Read the model definition and answer for the solid it produces. Units are mm, in the model's axes. A direction names the side the tool comes from. Give positions to 0.01 mm unless a question says otherwise; leave off trailing zeros. Order: outer loops, then holes, each group sorted by start corner. A loop starts at its lowest first (then second) coordinate and runs counter-clockwise, first axis right, second up. Notation, with made-up numbers: (38, 15.5) -> (88, 15.5) arc R23 cw to (88, 52.5) -> close; hole circle Ø5 at (60.25, 12.25). An arc over 180 degrees is marked (long way). Answer as CSV lines item,"result". Start each with the question number.
1) Straight lines are drawn through the part: L1, parallel to X at y = 7, z = -40; L2, parallel to X at y = 10, z = 10.25; L3, parallel to X at y = 1, z = -5. For each, find the intervals that lie inside material, in ascending order. Write a range as from..to.
2) Find section D-D (z = 7). Determine the outline of the cut face in (x, y), and give its area (3 significant figures).
3) The mould has two halves that part along Z. Classify faces 4 (the face through (82.4, 10.1, 8.2)), 5 (the face through (10, 70, 11.46)), 6 (the face through (62, 28, 5)), 7 (the face through (97, 5, -4)): +Z half, -Z half, draft (parallel to the pull), parting line (faces both ways), or undercut.
4) Find section A-A (z = -5). Determine the outline of the cut face in (x, y).
5) For faces 1 (the face through (3.659, 19.344, -1.767)), 2 (the face through (97, 2, -25)), 3 (the face through (87, 28, 5)), determine the directions among +Z, -Z, +X, -X, +Y, -Y from which every point of the face is accessible in a straight line to the end or side of a thin tool.
6) Find section B-B (x = 85). State how many separate pieces and enclosed holes the cut face has, and give its area (3 significant figures).
7) Flat-ended cylindrical pins translate along their axes: pin 1 Ø10 at (x, z) = (53, -17.5) entering from +Y; pin 2 Ø4 at (x, y) = (98, 3) entering from -Z; pin 3 Ø10 at (x, y) = (59.5, 28) entering from -Z. Find the tip coordinate at first contact, or state that the pin passes through.
```python
from build123d import *

# Parameters (mm, degrees)
BOSS_EXTRUDE1_DEPTH     = 10
SKETCH2_R               = 2.6
CUT_EXTRUDE1_DEPTH      = 142.774468788
BOSS_EXTRUDE3_START     = 10
SKETCH3_W               = 60
SKETCH3_H               = 9
SKETCH3_W_2             = 9
SKETCH3_H_2             = 60
BOSS_EXTRUDE3_DEPTH     = 1.46
CUT_EXTRUDE2_DEPTH      = 142.884923794
CUT_EXTRUDE2_DEPTH_BACK = 142.884923794
SKETCH2_2_R             = 2.6
CHAMFER1_SIZE           = 1.46
SKETCH4_R               = 4.5
CUT_EXTRUDE3_DEPTH      = 5
SKETCH5_W               = 100
SKETCH5_H               = 50
BOSS_EXTRUDE4_DEPTH     = 5
BOSS_EXTRUDE5_DEPTH     = 10
BOSS_EXTRUDE6_START     = 100
BOSS_EXTRUDE6_DEPTH     = 10
CUT_EXTRUDE4_DEPTH      = 151
CUT_EXTRUDE4_DEPTH_BACK = 151
SKETCH10_R              = 1.75
CUT_EXTRUDE5_START      = 100
SKETCH11_R              = 3.5
CUT_EXTRUDE5_DEPTH      = 95
SKETCH12_W              = 5
SKETCH12_H              = 10
SKETCH12_W_2            = 10
SKETCH12_H_2            = 5
CUT_EXTRUDE6_DEPTH      = 5
CHAMFER2_SIZE           = 5


# Some blends are built 0.0001 mm under size
with BuildPart() as part:
    # Sketch1 → Boss-Extrude1 (new body)
    with BuildSketch(Plane.XY):
        Polygon((0, 0), (100, 0), (100, 40), (20, 100), (0, 100), align=None)
    extrude(amount=BOSS_EXTRUDE1_DEPTH)

    # Sketch2 → Cut-Extrude1 (cut, through all)
    with BuildSketch(Plane.XY):
        with Locations((10, 85)):
            Circle(SKETCH2_R)
        with Locations((10, 60)):
            Circle(SKETCH2_R)
        with Locations((85, 30)):
            Circle(SKETCH2_R)
        with Locations((85, 10)):
            Circle(SKETCH2_R)
        with Locations((60, 10)):
            Circle(SKETCH2_R)
        with Locations((60, 30)):
            Circle(SKETCH2_R)
    extrude(amount=CUT_EXTRUDE1_DEPTH, mode=Mode.SUBTRACT)

    # Sketch3 → Boss-Extrude3 (add)
    with BuildSketch(Plane.XY.offset(BOSS_EXTRUDE3_START)):
        with Locations((70, 30)):
            Rectangle(SKETCH3_W, SKETCH3_H)
        with Locations((70, 10)):
            Rectangle(SKETCH3_W, SKETCH3_H)
        with Locations((10, 70)):
            Rectangle(SKETCH3_W_2, SKETCH3_H_2)
    extrude(amount=BOSS_EXTRUDE3_DEPTH)

    # Sketch2<2> → Cut-Extrude2 (cut, two sides: drawn at the far end of the back side and taken through both)
    with BuildSketch(Plane.XY.offset(-CUT_EXTRUDE2_DEPTH_BACK)):
        with Locations((10, 85)):
            Circle(SKETCH2_2_R)
        with Locations((10, 60)):
            Circle(SKETCH2_2_R)
        with Locations((85, 30)):
            Circle(SKETCH2_2_R)
        with Locations((85, 10)):
            Circle(SKETCH2_2_R)
        with Locations((60, 10)):
            Circle(SKETCH2_2_R)
        with Locations((60, 30)):
            Circle(SKETCH2_2_R)
    extrude(amount=CUT_EXTRUDE2_DEPTH + CUT_EXTRUDE2_DEPTH_BACK, mode=Mode.SUBTRACT)

    # Chamfer1
    chamfer1_edges = [part.edges().sort_by_distance(p)[0] for p in [
        (14.5, 70, 11.46),
        (5.5, 70, 11.46),
        (70, 5.5, 11.46),
        (70, 14.5, 11.46),
        (70, 25.5, 11.46),
        (70, 34.5, 11.46),
    ]]
    chamfer(chamfer1_edges, length=CHAMFER1_SIZE - 0.0001)  # a hair under: the kernel refuses the full size

    # Sketch4 → Cut-Extrude3 (cut)
    with BuildSketch(Plane.XY):
        with Locations((10, 85)):
            Circle(SKETCH4_R)
        with Locations((10, 60)):
            Circle(SKETCH4_R)
        with Locations((60, 30)):
            Circle(SKETCH4_R)
        with Locations((85, 30)):
            Circle(SKETCH4_R)
        with Locations((85, 10)):
            Circle(SKETCH4_R)
        with Locations((60, 10)):
            Circle(SKETCH4_R)
    extrude(amount=CUT_EXTRUDE3_DEPTH, mode=Mode.SUBTRACT)

    # Sketch5 → Boss-Extrude4 (add)
    with BuildSketch(Plane(origin=(0, 0, 0), x_dir=(1, 0, 0), z_dir=(0, 1, 0))):
        with Locations((50, 25)):
            Rectangle(SKETCH5_W, SKETCH5_H)
    extrude(amount=BOSS_EXTRUDE4_DEPTH)

    # Sketch8 → Boss-Extrude5 (add)
    with BuildSketch(Plane(origin=(0, 0, 0), x_dir=(0, 0, -1), z_dir=(1, 0, 0))):
        Polygon((-10, 5), (50, 5), (-10, 40), align=None)
    extrude(amount=BOSS_EXTRUDE5_DEPTH)

    # Sketch8<2> → Boss-Extrude6 (add)
    with BuildSketch(Plane(origin=(0, 0, 0), x_dir=(0, 0, -1), z_dir=(1, 0, 0)).offset(BOSS_EXTRUDE6_START)):
        Polygon((-10, 5), (50, 5), (-10, 40), align=None)
    extrude(amount=-BOSS_EXTRUDE6_DEPTH)

    # Sketch10 → Cut-Extrude4 (cut, two sides: drawn at the far end of the back side and taken through both)
    with BuildSketch(Plane(origin=(0, 0, 0), x_dir=(1, 0, 0), z_dir=(0, 1, 0)).offset(-CUT_EXTRUDE4_DEPTH_BACK)):
        with Locations(Location((5, 40, 0), (0, 0, 90))):
            Circle(SKETCH10_R)
        with Locations(Location((95, 40, 0), (0, 0, 90))):
            Circle(SKETCH10_R)
        with Locations(Location((95, 5, 0), (0, 0, 90))):
            Circle(SKETCH10_R)
        with Locations(Location((5, 5, 0), (0, 0, 90))):
            Circle(SKETCH10_R)
    extrude(amount=CUT_EXTRUDE4_DEPTH + CUT_EXTRUDE4_DEPTH_BACK, mode=Mode.SUBTRACT)

    # Sketch11 → Cut-Extrude5 (cut)
    with BuildSketch(Plane(origin=(0, 0, 0), x_dir=(1, 0, 0), z_dir=(0, 1, 0)).offset(CUT_EXTRUDE5_START)):
        with Locations(Location((5, 5, 0), (0, 0, 270))):
            Circle(SKETCH11_R)
        with Locations(Location((5, 40, 0), (0, 0, 270))):
            Circle(SKETCH11_R)
        with Locations(Location((95, 40, 0), (0, 0, 270))):
            Circle(SKETCH11_R)
        with Locations(Location((95, 5, 0), (0, 0, 270))):
            Circle(SKETCH11_R)
    extrude(amount=-CUT_EXTRUDE5_DEPTH, mode=Mode.SUBTRACT)

    # Sketch12 → Cut-Extrude6 (cut)
    with BuildSketch(Plane(origin=(0, 0, 0), x_dir=(1, 0, 0), z_dir=(0, 1, 0))):
        with Locations((97.5, 20)):
            Rectangle(SKETCH12_W, SKETCH12_H)
        with Locations((2.5, 20)):
            Rectangle(SKETCH12_W, SKETCH12_H)
        with Locations((50, 47.5)):
            Rectangle(SKETCH12_W_2, SKETCH12_H_2)
    extrude(amount=CUT_EXTRUDE6_DEPTH, mode=Mode.SUBTRACT)

    # Chamfer2
    # the kernel refuses this chamfer: 5 mm, written as the material it takes off along each edge
    with BuildSketch(Plane(origin=(3.333333333, 96.666666667, 3.333333333), x_dir=(0.7071067811865475, 0.7071067811865476, 0), z_dir=(-0.5773502691896258, 0.5773502691896258, -0.5773502691896258))) as chamfer2_piece_1:
        Polygon((-3.535533906, -2.041241452), (3.535533906, -2.041241452), (0, 4.082482905), align=None)
    extrude(amount=6.350852961, mode=Mode.SUBTRACT)
    with BuildSketch(Plane(origin=(100, -12.85841494, -50), x_dir=(0.0274958766105877, 0, 0.9996219169112968), z_dir=(0, 1, 0))) as chamfer2_piece_2:
        Polygon((CHAMFER2_SIZE * 0.999621916911, -CHAMFER2_SIZE * 0.0274958766106), (-CHAMFER2_SIZE * 0.0274958766106, -CHAMFER2_SIZE * 0.999621916911), (0, 0), align=None)
    extrude(amount=30.71682988, mode=Mode.SUBTRACT)
    with BuildSketch(Plane(origin=(0, -12.85841494, -50), x_dir=(-0.027495876610586372, 0, 0.9996219169112968), z_dir=(0, 1, 0))) as chamfer2_piece_3:
        Polygon((CHAMFER2_SIZE * 0.999621916911, CHAMFER2_SIZE * 0.0274958766106), (-CHAMFER2_SIZE * 0.0274958766106, CHAMFER2_SIZE * 0.999621916911), (0, 0), align=None)
    extrude(amount=30.71682988, mode=Mode.SUBTRACT)
    with BuildSketch(Plane(origin=(0, 100, -12.85841494), x_dir=(0.9996219169112968, 0.0274958766105877, 0), z_dir=(0, 0, 1))) as chamfer2_piece_4:
        Polygon((CHAMFER2_SIZE * 0.999621916911, -CHAMFER2_SIZE * 0.0274958766106), (-CHAMFER2_SIZE * 0.0274958766106, -CHAMFER2_SIZE * 0.999621916911), (0, 0), align=None)
    extrude(amount=35.71682988, mode=Mode.SUBTRACT)
    with BuildSketch(Plane(origin=(110.286731952, 32.284951036, 0), x_dir=(0.016497525966350957, 0.021996701288467948, 0.9996219169112968), z_dir=(-0.8000000000000002, 0.6, 0))) as chamfer2_piece_5_section:
        Polygon((CHAMFER2_SIZE * 0.999621916911, -CHAMFER2_SIZE * 0.0274958766106), (-CHAMFER2_SIZE * 0.0274958766106, -CHAMFER2_SIZE * 0.999621916911), (0, 0), align=None)
    chamfer2_piece_5 = extrude(amount=125.71682988, mode=Mode.PRIVATE)
    chamfer2_piece_5 = split(chamfer2_piece_5, bisect_by=Plane(origin=(58.587038142, 43.71482671, 16.368274359), z_dir=(0, 0.8637789008984335, -0.5038710255240861)), keep=Keep.TOP, mode=Mode.PRIVATE)
    add(chamfer2_piece_5, mode=Mode.SUBTRACT)
    with BuildSketch(Plane(origin=(32.85841494, 100, 0), x_dir=(0, 0.0274958766105877, 0.9996219169112968), z_dir=(-1, 0, 0))) as chamfer2_piece_6:
        Polygon((CHAMFER2_SIZE * 0.999621916911, -CHAMFER2_SIZE * 0.0274958766106), (-CHAMFER2_SIZE * 0.0274958766106, -CHAMFER2_SIZE * 0.999621916911), (0, 0), align=None)
    extrude(amount=45.71682988, mode=Mode.SUBTRACT)
    with BuildSketch(Plane(origin=(0, 112.85841494, 0), x_dir=(-0.02749587661058638, 0, 0.9996219169112968), z_dir=(0, -1, 0))) as chamfer2_piece_7_section:
        Polygon((CHAMFER2_SIZE * 0.999621916911, -CHAMFER2_SIZE * 0.0274958766106), (-CHAMFER2_SIZE * 0.0274958766106, -CHAMFER2_SIZE * 0.999621916911), (0, 0), align=None)
    chamfer2_piece_7 = extrude(amount=91.550163213, mode=Mode.PRIVATE)
    chamfer2_piece_7 = split(chamfer2_piece_7, bisect_by=Plane(origin=(1.672912206, 43.366191756, 15.770614439), z_dir=(0, 0.8637789008984335, -0.5038710255240861)), keep=Keep.TOP, mode=Mode.PRIVATE)
    add(chamfer2_piece_7, mode=Mode.SUBTRACT)


solid = part.part
```
Findings below:
1,L1,"0..1.5, 8.5..10, 90..91.5, 98.5..100"
1,L2,"40..57.4, 62.6..82.4, 87.6..100"
1,L3,"0..3.25, 6.75..93.25, 96.75..100"
2,outline,"(0, 0) -> (100, 0) -> (100, 40) -> (20, 100) -> (5, 100) -> (0, 95) -> close; hole circle Ø5.2 at (10, 60); hole circle Ø5.2 at (10, 85); hole circle Ø5.2 at (60, 10); hole circle Ø5.2 at (60, 30); hole circle Ø5.2 at (85, 10); hole circle Ø5.2 at (85, 30)"
2,area,"7,460 mm²"
3,face 4,"draft"
3,face 5,"+Z half"
3,face 6,"-Z half"
3,face 7,"undercut"
4,outline,"(0, 0) -> (3.25, 0) -> (3.25, 5) -> (1.5, 5) -> (1.5, 31.25) -> (0, 31.25) -> close; (6.75, 0) -> (93.25, 0) -> (93.25, 5) -> (91.5, 5) -> (91.5, 31.25) -> (90, 31.25) -> (90, 5) -> (10, 5) -> (10, 31.25) -> (8.5, 31.25) -> (8.5, 5) -> (6.75, 5) -> close; (96.75, 0) -> (100, 0) -> (100, 31.25) -> (98.5, 31.25) -> (98.5, 5) -> (96.75, 5) -> close"
5,face 1,"+Y"
5,face 2,"+X, -Y"
5,face 3,"-Z"
6,separate pieces,"3"
6,enclosed holes,"0"
6,area,"612 mm²"
7,pin 1,"y = 5"
7,pin 2,"z = -49"
7,pin 3,"z = 0"
